Can you work these out from the model? Positions are in its coordinate system, mm. A direction names the side the tool comes from. Give positions to 0.01 mm unless a question says otherwise; leave off trailing zeros. Loops run counter-clockwise (first coordinate to the right, second up) from the corner with the lowest first, then second, coordinate; pieces in that order, holes last. Notation, with made-up numbers: M 33,35.25 L 60,35.25 A25 ccw 60,52.25 Z; hole C 22.5,6.5 d6. An arc over 180 degrees is marked long. Put each result on its own line as item: value. Start each with the question number.
1) Imagine slicing it at C-C (y = 92.5). Write out the boundary of the cut face in (x, z), then the cut area to 3 significant figures.
2) Imagine slicing it at A-A (x = -10). Write out the boundary of the cut face in (y, z) (3 decimals).
3) For faces 1 (the flat face through (0, 390.009, -30)), 2 (the flat face through (0, 383.699, -27)), which set-ups out of +Z, -Z, +X, -X, +Y, -Y let a thin tool reach every point of the face, with its end or its side?
4) For P1, Ø1, axis at x = 2, z = 39, coming from the -Y side; P2, Ø19, axis at x = 0.5, y = 212, coming from the +Z side, each with a flat end and sliding along its axis, tell me the tip position at first contact or that it passes through.
5) Please list where these lines run through material, in increasing order: line 1 along Z through (x, y) = (8.5, -28); line 2 along Y through (x, z) = (4.5, 122.5). Write a range as from..to.
6) Imagine slicing it at B-B (z = -51). Write out the boundary of the cut face in (x, y), then the cut area to 3 significant figures.
from build123d import *

# Parameters (mm, degrees)
CROQUIS1_W              = 38.1
CROQUIS1_H              = 850.5
SALIENTE_EXTRUIR1_DEPTH = 6.31
CROQUIS2_W              = 38.1
CROQUIS2_H              = 6.31
SALIENTE_EXTRUIR2_DEPTH = 70
CROQUIS3_W              = 38.1
CROQUIS3_H              = 6.31
SALIENTE_EXTRUIR3_DEPTH = 578
CROQUIS4_R              = 6.935856655
CORTAR_EXTRUIR1_DEPTH   = 7
CROQUIS5_W              = 38.1
CROQUIS5_H              = 687.72607772
CORTAR_EXTRUIR2_DEPTH   = 10
CROQUIS6_W              = 38.1
CROQUIS6_H              = 6.31
CROQUIS8_W              = 368.89
CROQUIS8_H              = 6.31
CORTAR_EXTRUIR3_DEPTH   = 147


with BuildPart() as part:
    # Croquis1 → Saliente-Extruir1 (new body)
    with BuildSketch(Plane.XY):
        Rectangle(CROQUIS1_W, CROQUIS1_H)
    extrude(amount=SALIENTE_EXTRUIR1_DEPTH)

    # Croquis2 → Saliente-Extruir2 (add)
    with BuildSketch(Plane.XY.offset(6.31)):
        with Locations((0, -422.095)):
            Rectangle(CROQUIS2_W, CROQUIS2_H)
    extrude(amount=SALIENTE_EXTRUIR2_DEPTH)

    # Croquis3 → Saliente-Extruir3 (add)
    with BuildSketch(Plane.XY.offset(6.31)):
        with Locations((0, -265.63107772)):
            Rectangle(CROQUIS3_W, CROQUIS3_H)
    extrude(amount=-SALIENTE_EXTRUIR3_DEPTH)

    # Croquis4 → Cortar-Extruir1 (cut)
    with BuildSketch(Plane(origin=(0, -262.47607772, 0), x_dir=(1, 0, 0), z_dir=(0, 1, 0))):
        with Locations(Location((0, 536.981534281, 0), (0, 0, 270))):
            Circle(CROQUIS4_R)
    extrude(amount=-CORTAR_EXTRUIR1_DEPTH, mode=Mode.SUBTRACT)

    # Croquis5 → Cortar-Extruir2 (cut)
    with BuildSketch(Plane(origin=(0, 0, 0), x_dir=(-1, 0, 0), z_dir=(0, 0, -1))):
        with Locations((0, 81.38696114)):
            Rectangle(CROQUIS5_W, CROQUIS5_H)
    extrude(amount=-CORTAR_EXTRUIR2_DEPTH, mode=Mode.SUBTRACT)

    # Barrer1: sweep along a curve in space
    with BuildLine() as barrer1_path:
        Line((0, -262.47607772, -199.645), (0, 386.85392228, -199.645))
        Line((0, 386.85392228, -199.645), (0, 386.85392228, 137.595))
    # Croquis6 → Barrer1 (sweep)
    with BuildSketch(Plane(origin=(0, -262.47607772, 0), x_dir=(1, 0, 0), z_dir=(0, 1, 0))):
        with Locations((0, 199.645)):
            Rectangle(CROQUIS6_W, CROQUIS6_H)
    sweep(path=barrer1_path.line, transition=Transition.RIGHT)

    # Croquis8 → Cortar-Extruir3 (cut)
    with BuildSketch(Plane(origin=(19.05, 0, 0), x_dir=(0, 0, -1), z_dir=(1, 0, 0))):
        Polygon((196.49, -262.47607772), (196.49, -268.78607772), (196.49, -444.307673596), (-90.834600665, -444.307673596), (-90.834600665, -262.47607772), align=None)
        with Locations((387.245, -265.63107772)):
            Rectangle(CROQUIS8_W, CROQUIS8_H)
    extrude(amount=-CORTAR_EXTRUIR3_DEPTH, mode=Mode.SUBTRACT)


solid = part.part
Recorded:
1. outline: M -19.05,-202.8 L 19.05,-202.8 L 19.05,-196.49 L -19.05,-196.49 Z
1. area: 240 mm²
2. outline: M -268.786,-202.8 L 390.009,-202.8 L 390.009,137.595 L 383.699,137.595 L 383.699,-196.49 L -268.786,-196.49 Z
3. face 1: +Z, -Z, +X, -X, +Y
3. face 2: +Z, +X, -X, -Y
4. P1: y = 383.7
4. P2: z = -196.49
5. line 1: -202.8..-196.49
5. line 2: 383.7..390.01
6. outline: M -19.05,383.7 L 19.05,383.7 L 19.05,390.01 L -19.05,390.01 Z
6. area: 240 mm²
